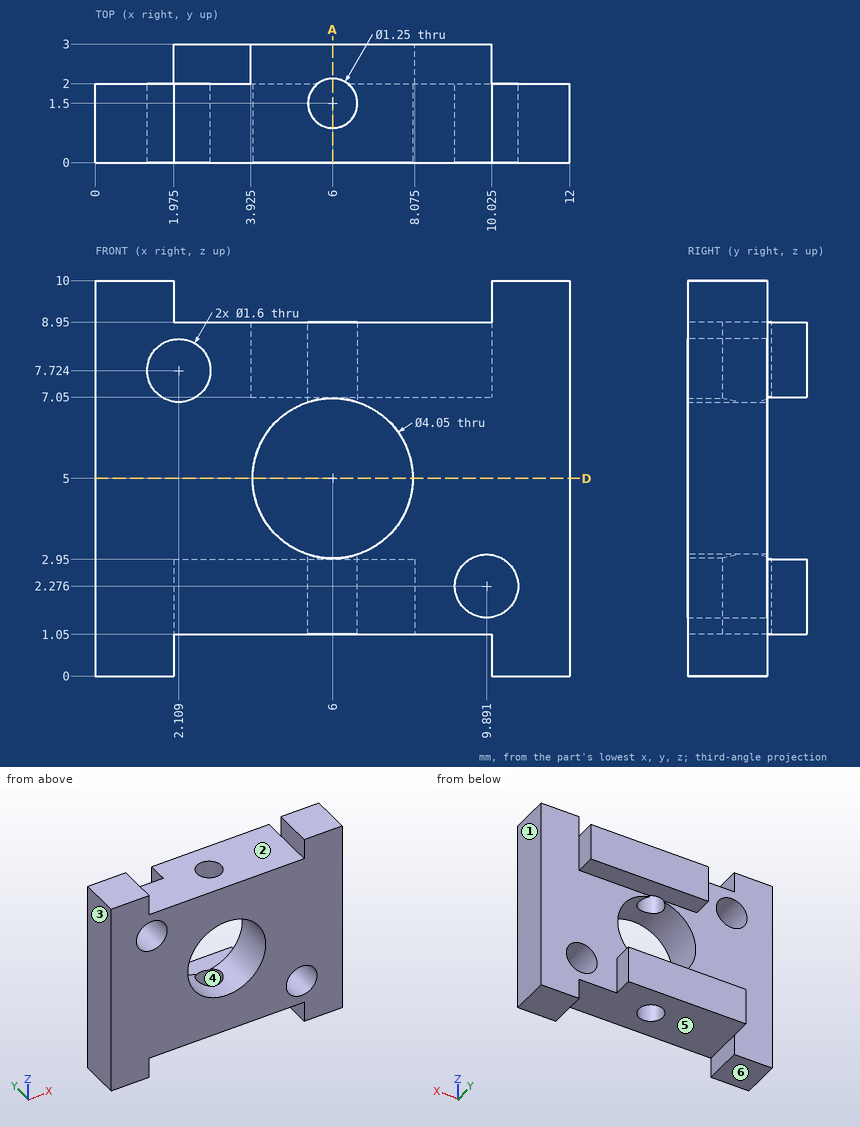
Answer from the drawing. Dimensions are ordinates in mm from the lowest x, y and z of the part. A direction names the side the tool comes from. Round coordinates to 2 decimals unless told otherwise and drop trailing zeros. Write each loop counter-clockwise with the first axis right and the second up, starting at its lowest first coordinate (ties: lowest second). Pieces come first, ordered by that corner, then holes. Notation, with made-up numbers: (-23, 10.25) -> (2, 10.25) arc R11 ccw to (2, 29.25) -> close; hole circle Ø9 at (54, 10.25). An arc over 180 degrees is marked (long way). Write each question's results on one line, items separated by ' | '.
1) The part is cut by section A-A (x = 6). State how many separate pieces and enclosed holes the cut face has.
Findings:
separate pieces: 4 | enclosed holes: 0
2) Which of the six approach directions +Z, -Z, +X, -X, +Y, -Y give full straight-line access (tool end or side, diameter ignored) to the marked faces 5 and 6?
Findings:
face 5: -Z, +Y, -Y | face 6: -Z, +X, -X, +Y, -Y
3) For a pull along X with two mould halves and no side action, classify the marked faces 1, 2, 3 and 4 as +X half, -X half, draft (parallel to the pull), parting line (faces both ways), or undercut.
Findings:
face 1: +X half | face 2: undercut | face 3: -X half | face 4: undercut
4) The part is cut by section D-D (z = 5). Write down the section's boundary in (x, y) (1 decimal).
Findings:
outline: (0, 0) -> (4, 0) -> (4, 2) -> (0, 2) -> close; (8, 0) -> (12, 0) -> (12, 2) -> (8, 2) -> close
5) Flat-ended cylindrical pins translate along their axes: pin 1 (1.5 mm diameter, centred on x = 4.5, y = 1.5, fed in from -Z); pin 2 (2 mm diameter, centred on x = 2.11, z = 7.72, fed in from +Y); pin 3 (1.1 mm diameter, centred on x = 6, y = 1.5, fed in from +Z); pin 4 (1.1 mm diameter, centred on x = 4, y = 2.5, fed in from +Z). Find the tip coordinate at first contact, or state that the pin passes through.
Findings:
pin 1: stops at z = 1.05 | pin 2: stops at y = 2 | pin 3: passes through | pin 4: stops at z = 8.95
6) Consider line 1 along X through (y, z) = (1.85, 9) (1 decimal); line 2 along Z through (x, y) = (4.5, 2.35); line 3 along Y through (x, z) = (1.5, 9.75). Determine where each line is inside the solid, lowest interval first. Write a range as [from, to].
Findings:
line 1: x = [0, 2], [10, 12] | line 2: z = [1.05, 2.95], [7.05, 8.95] | line 3: y = [0, 2]
